```python
from build123d import *

# Parameters (mm, degrees)
SKETCH1_R           = 1.5
BOSS_EXTRUDE1_DEPTH = 4
SKETCH2_R           = 7.5
BOSS_EXTRUDE2_DEPTH = 5.5


with BuildPart() as part:
    # Sketch1 → Boss-Extrude1 (new body)
    with BuildSketch(Plane(origin=(0, 0, 0), x_dir=(1, 0, 0), z_dir=(0, 1, 0))):
        with BuildLine():
            Line((-19, 16.248076809), (-19, -16.248076809))
            ThreePointArc((-19, -16.248076809), (25, 0), (-19, 16.248076809))
        make_face()
        with Locations(Location((12.5, 12.5, 0), (0, 0, 270))):
            Circle(SKETCH1_R, mode=Mode.SUBTRACT)
        with Locations(Location((12.5, -12.5, 0), (0, 0, 270))):
            Circle(SKETCH1_R, mode=Mode.SUBTRACT)
        with Locations(Location((-12.5, -12.5, 0), (0, 0, 270))):
            Circle(SKETCH1_R, mode=Mode.SUBTRACT)
        with Locations(Location((-12.5, 12.5, 0), (0, 0, 270))):
            Circle(SKETCH1_R, mode=Mode.SUBTRACT)
        with BuildLine():
            Line((-1.5, 2.598076211), (-1.5, -2.598076211))
            ThreePointArc((-1.5, -2.598076211), (3, 0), (-1.5, 2.598076211))
        make_face(mode=Mode.SUBTRACT)
    extrude(amount=BOSS_EXTRUDE1_DEPTH)

    # Sketch2 → Boss-Extrude2 (add)
    with BuildSketch(Plane(origin=(0, 4, 0), x_dir=(1, 0, 0), z_dir=(0, 1, 0))):
        with Locations(Location((0, 0, 0), (0, 0, 270))):
            Circle(SKETCH2_R)
        with BuildLine():
            Line((-1.5, 2.598076211), (-1.5, -2.598076211))
            ThreePointArc((-1.5, -2.598076211), (3, 0), (-1.5, 2.598076211))
        make_face(mode=Mode.SUBTRACT)
    extrude(amount=BOSS_EXTRUDE2_DEPTH)


solid = part.part
```
The listing builds one solid part. Answer for the finished solid, in the listing's coordinates (mm). A direction names the side the tool comes from. Give positions to 0.01 mm unless a question says otherwise; leave off trailing zeros. Loops run counter-clockwise (first coordinate to the right, second up) from the corner with the lowest first, then second, coordinate; pieces in that order, holes last. Notation, with made-up numbers: M -28,88 L -17,88 A30 ccw -17,116 Z; hole C 52.5,75.25 d1. An arc over 180 degrees is marked long. One line per item, written item: value.
Q1. For faces 1 (the face through (-2, 9.5, 0)), 2 (the face through (-1.5, 5, 0)), 3 (the face through (0.33, 6.712, -7.493)), determine the directions among +Z, -Z, +X, -X, +Y, -Y from which every point of the face is accessible in a straight line to the end or side of a thin tool.
Working result:
face 1: +Z, -Z, +X, -X, +Y
face 2: +Y, -Y
face 3: +Y
Q2. A cutting plane is placed at D-D on z = 0. Determine the outline of the cut face in (x, y), then the cut area to 3 significant figures.
Working result:
outline: M -19,0 L -1.5,0 L -1.5,9.5 L -7.5,9.5 L -7.5,4 L -19,4 Z; M 3,0 L 25,0 L 25,4 L 7.5,4 L 7.5,9.5 L 3,9.5 Z
area: 216 mm^2
Q3. Determine the mould class of faces 4 (the face through (-12.43, 1.97, 11)), 5 (the face through (-2, 0, 0)), 6 (the face through (24.985, 1.972, 0.852)) for opening direction Z: +Z half, -Z half, draft (parallel to the pull), parting line (faces both ways), or undercut.
Working result:
face 4: undercut
face 5: draft
face 6: parting line
Q4. Find the intervals of material crossed by line 1 (Z direction, x = 0, y = 2.5); line 2 (X direction, y = 3.2, z = 12.5); line 3 (Y direction, x = -7, z = 17), in increasing order. Write a range as from..to.
Working result:
line 1: z = -25..-3, 3..25
line 2: x = -19..-14, -11..11, 14..21.65
line 3: y = 0..4
Q5. A cutting plane is placed at C-C on x = -12.5. Determine the outline of the cut face in (y, z), then the cut area to 3 significant figures.
Working result:
outline: M 0,-21.65 L 4,-21.65 L 4,-14 L 0,-14 Z; M 0,-11 L 4,-11 L 4,11 L 0,11 Z; M 0,14 L 4,14 L 4,21.65 L 0,21.65 Z
area: 149 mm^2
Q6. A cutting plane is placed at B-B on z = -12.5. Determine the outline of the cut face in (x, y).
Working result:
outline: M -19,0 L -14,0 L -14,4 L -19,4 Z; M -11,0 L 11,0 L 11,4 L -11,4 Z; M 14,0 L 21.65,0 L 21.65,4 L 14,4 Z
Q7. Flat-ended cylindrical pins translate along their axes: P1, Ø1.5, axis at x = 19, z = -9, coming from the -Y side; P2, Ø4, axis at x = 13.5, y = 1.5, coming from the -Z side; P3, Ø4, axis at y = 4, z = 0, coming from the +X side; P4, Ø6, axis at x = 17, z = 5.5, coming from the +Y side. Find the tip coordinate at first contact, or state that the pin passes through.
Working result:
P1: stops at y = 0
P2: stops at z = -22.2
P3: stops at x = 25
P4: stops at y = 4
Q8. A cutting plane is placed at A-A on x = 0. Determine the outline of the cut face in (y, z), then the cut area to 4 significant figures.
Working result:
outline: M 0,-25 L 4,-25 L 4,-7.5 L 9.5,-7.5 L 9.5,-3 L 0,-3 Z; M 0,3 L 9.5,3 L 9.5,7.5 L 4,7.5 L 4,25 L 0,25 Z
area: 225.5 mm^2
